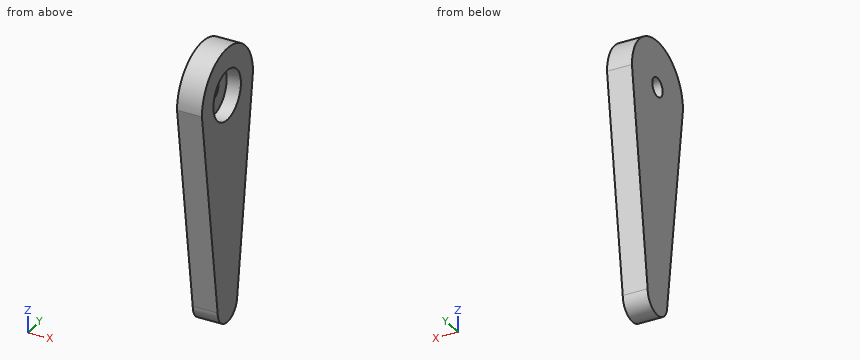
```python
from build123d import *

# Parameters (mm, degrees)
CYLINDER_R     = 7
CYLINDER_DEPTH = 5
SKETCH_R       = 2.644595
PAD_DEPTH      = 7


with BuildPart() as cylinder:
    # Cylinder → Cylinder (new body)
    with BuildSketch(Plane(origin=(13.5, 25, 39), x_dir=(0, 0, -1), z_dir=(1, 0, 0))):
        Circle(CYLINDER_R)
    extrude(amount=CYLINDER_DEPTH)


with BuildPart() as cut:
    # Sketch → Pad (new body)
    with BuildSketch(Plane.YZ):
        with BuildLine():
            Line((12.552548, 39.037066), (20.552548, -20.427209))
            ThreePointArc((20.552548, -20.427209), (25.552548, -25.427189), (30.552548, -20.427209))
            Line((30.552548, -20.427209), (38.552548, 39.037066))
            ThreePointArc((38.552548, 39.037066), (25.552548, 52.03702), (12.552548, 39.037066))
        make_face()
        with Locations((25.552548, 39.03702)):
            Circle(SKETCH_R, mode=Mode.SUBTRACT)
    extrude(amount=PAD_DEPTH)


with BuildPart() as cut_1:
    # Body placement: moved
    add(cut.part.moved(Location((10.5, -0.4, 0.2))))

    # Cut: cut Cylinder
    add(cylinder.part, mode=Mode.SUBTRACT)


solid = cut_1.part
```
Could you check a few things on this model? Use its own coordinates, in mm. Round coordinates to 2 decimals unless told otherwise and drop trailing zeros. Loops run counter-clockwise (first coordinate to the right, second up) from the corner with the lowest first, then second, coordinate; pieces in that order, holes last. Notation, with made-up numbers: (62, -10.5) -> (111, -10.5) arc R13 ccw to (111, 6.5) -> close; hole circle Ø6 at (17, 2). An arc over 180 degrees is marked (long way). Put each result on its own line as item: value.
Q1. For pin 1 Ø4 at (y, z) = (24, 37) entering from +X; pin 2 Ø1 at (x, z) = (13, 36) entering from +Y; pin 3 Ø2 at (x, y) = (16, 22) entering from +Z, each with a flat end and sliding along its axis, tell me the tip position at first contact or that it passes through.
Checks:
pin 1: x = 13.5
pin 2: y = 37.78
pin 3: z = 52.06
Q2. Please list where these lines run through material, in increasing order: line 1 (Z direction, x = 16.5, y = 25); line 2 (Y direction, x = 14.5, z = 36.5); line 3 (Z direction, x = 12, y = 24.75). Write a range as from..to.
Checks:
line 1: -25.22..32, 46..52.24
line 2: 12.52..18.46, 31.54..37.78
line 3: -25.21..36.62, 41.85..52.23
Q3. I want a section at B-B on x = 14.75. Write out the boundary of the cut face in (y, z), and give its area (3 significant figures).
Checks:
outline: (12.15, 39.24) -> (20.15, -20.23) arc R5 ccw to (30.15, -20.23) -> (38.15, 39.24) arc R13 ccw to start; hole circle Ø14 at (25, 39)
area: 1,220 mm2
Q4. I want a section at D-D on z = 14. Write out the boundary of the cut face in (x, y), and give its area (3 significant figures).
Checks:
outline: (10.5, 15.55) -> (17.5, 15.55) -> (17.5, 34.76) -> (10.5, 34.76) -> close
area: 134 mm2
Q5. I want a section at A-A on y = 26.75. Write out the boundary of the cut face in (x, z), and give its area (3 significant figures).
Checks:
outline: (10.5, -24.97) -> (17.5, -24.97) -> (17.5, 32.22) -> (13.5, 32.22) -> (13.5, 37.13) -> (10.5, 37.13) -> close; (10.5, 41.34) -> (13.5, 41.34) -> (13.5, 45.78) -> (17.5, 45.78) -> (17.5, 52.14) -> (10.5, 52.14) -> close
area: 473 mm2
Q6. I want a section at C-C on y = 34.25. Write out the boundary of the cut face in (x, z).
Checks:
outline: (10.5, 10.23) -> (17.5, 10.23) -> (17.5, 48.52) -> (10.5, 48.52) -> close
